Can you work these out from the model? Positions are in its coordinate system, mm. A direction names the side the tool comes from. Round coordinates to 2 decimals unless told otherwise and drop trailing zeros. Loops run counter-clockwise (first coordinate to the right, second up) from the corner with the lowest first, then second, coordinate; pieces in that order, holes last. Notation, with made-up numbers: (43.5, -29.75) -> (50.5, -29.75) arc R6 cw to (50.5, -20.75) -> close; hole circle Ø8 at (6, -12.75). An arc over 180 degrees is marked (long way). Write item = value, one per line.
from build123d import *

# Parameters (mm, degrees)
F0_W      = 101.6
F0_H      = 101.6
F1_DEPTH  = 80.01
F2_R      = 25.4
F1_FACE_W = 50.8
F1_FACE_H = 50.8
F3_DEPTH  = 50.8


with BuildPart() as f1:
    # F0 (on Top) → F1 (new body)
    with BuildSketch(Plane.XY):
        with Locations((17.88482, 13.020775)):
            Rectangle(F0_W, F0_H)
    extrude(amount=F1_DEPTH)

    # F2
    f2_edges = [f1.edges().sort_by_distance(p)[0] for p in [
        (17.88482, -37.779225, 80.01),
        (-32.91518, 13.020775, 80.01),
        (17.88482, 63.820775, 80.01),
        (68.68482, 13.020775, 80.01),
    ]]
    fillet(f2_edges, radius=F2_R)

    # F1_face (on face) → F3 (join)
    with BuildSketch(Plane(origin=(17.88482, 13.020775, 80.01), x_dir=(1, 0, 0), z_dir=(0, 0, 1))):
        Rectangle(F1_FACE_W, F1_FACE_H)
    extrude(amount=F3_DEPTH)


solid = f1.part
1. I need wall thicknesses on line 1 (Y direction, x = 10, z = 116.5); line 2 (Y direction, x = -5.5, z = 62.5); line 3 (X direction, y = 13, z = 109). Which ranges of each line are inside material? Lowest first, please. Write a range as [from, to].
Entries:
line_1 = [-12.38, 38.42]
line_2 = [-36.52, 62.56]
line_3 = [-7.52, 43.28]
2. I'm going to push a flat-ended pin straight in: pin 1 (2 mm diameter, centred on y = 35.5, z = 79, fed in from +X). Where does the tip first touch, or does it pass through?
Entries:
pin_1 = 53.19
3. Suppose I cut it at A-A, the plane x = 12. List the corners of the cut face in (y, z) for me.
Entries:
outline = (-37.78, 0) -> (63.82, 0) -> (63.82, 54.61) arc R25.4 ccw to (38.42, 80.01) -> (38.42, 130.81) -> (-12.38, 130.81) -> (-12.38, 80.01) arc R25.4 ccw to (-37.78, 54.61) -> close
4. Suppose I cut it at B-B, the plane y = 1. List the corners of the cut face in (x, z) for me.
Entries:
outline = (-32.92, 0) -> (68.68, 0) -> (68.68, 54.61) arc R25.4 ccw to (43.28, 80.01) -> (43.28, 130.81) -> (-7.52, 130.81) -> (-7.52, 80.01) arc R25.4 ccw to (-32.92, 54.61) -> close
5. For faces 1 (the flat face through (-7.515, 13, 105)), 2 (the flat face through (18, -12.379, 105)), 3 (the flat face through (43.285, 13, 105)), which set-ups out of +Z, -Z, +X, -X, +Y, -Y let a thin tool reach every point of the face, with its end or its side?
Entries:
face_1 = +Z, -X, +Y, -Y
face_2 = +Z, +X, -X, -Y
face_3 = +Z, +X, +Y, -Y
6. Suppose I cut it at C-C, the plane z = 93. List the corners of the cut face in (x, y) for me.
Entries:
outline = (-7.52, -12.38) -> (43.28, -12.38) -> (43.28, 38.42) -> (-7.52, 38.42) -> close
7. Suppose I cut it at D-D, the plane y = -24.5. List the corners of the cut face in (x, z) for me.
Entries:
outline = (-32.92, 0) -> (68.68, 0) -> (68.68, 54.61) arc R25.4 ccw to (55.41, 76.93) -> (-19.64, 76.93) arc R25.4 ccw to (-32.92, 54.61) -> close
